from build123d import *

# Parameters (mm, degrees)
BOSS_EXTRUDE1_DEPTH                                 = 12
SHELL1_T                                            = -2.5
FILLET2_R                                           = 8
SKETCH5_R                                           = 1.5
BOSS_EXTRUDE3_DEPTH                                 = 9.5
FILLET5_R                                           = 4
CSK_FOR_M4_COUNTERSUNK_FLAT_HEAD_SCREW1_D           = 4.5
CSK_FOR_M4_COUNTERSUNK_FLAT_HEAD_SCREW1_CSINK_D     = 9.4
CSK_FOR_M4_COUNTERSUNK_FLAT_HEAD_SCREW1_CSINK_ANGLE = 90
CSK_FOR_M4_COUNTERSUNK_FLAT_HEAD_SCREW2_D           = 4.5
CSK_FOR_M4_COUNTERSUNK_FLAT_HEAD_SCREW2_CSINK_D     = 9.4
CSK_FOR_M4_COUNTERSUNK_FLAT_HEAD_SCREW2_CSINK_ANGLE = 90


with BuildPart() as part:
    # Sketch1 → Boss-Extrude1 (new body)
    with BuildSketch(Plane.XZ.offset(-76.724152422)):
        with BuildLine():
            Line((110.259063934, 82.346126643), (10.232808146, 82.346126643))
            ThreePointArc((10.232808146, 82.346126643), (4.41063977, 84.859565296), (2.246887156, 90.820537791))
            Line((2.246887156, 90.820537791), (13.35579753, 277.820529099))
            ThreePointArc((13.35579753, 277.820529099), (15.855157174, 283.168286326), (21.341718521, 285.346117951))
            Line((21.341718521, 285.346117951), (99.259600005, 285.346117951))
            ThreePointArc((99.259600005, 285.346117951), (104.747858971, 283.166686096), (107.245796332, 277.815871333))
            Line((107.245796332, 277.815871333), (118.24526026, 90.815880025))
            ThreePointArc((118.24526026, 90.815880025), (116.079632079, 84.857867678), (110.259063934, 82.346126643))
        make_face()
    extrude(amount=BOSS_EXTRUDE1_DEPTH)

    # Shell1
    shell1_openings = [part.faces().sort_by_distance(p)[0] for p in [
        (60.272055657, 76.724152422, 180.004596884),
    ]]
    offset(amount=SHELL1_T, openings=shell1_openings, kind=Kind.INTERSECTION)

    # Fillet2
    fillet2_edges = [part.edges().sort_by_distance(p)[0] for p in [
        (104.747858971, 64.724152422, 283.166686096),
        (60.300659263, 64.724152422, 285.346117951),
        (15.855157174, 64.724152422, 283.168286326),
        (7.801342343, 64.724152422, 184.320533445),
        (4.41063977, 64.724152422, 84.859565296),
        (60.24593604, 64.724152422, 82.346126643),
        (116.079632079, 64.724152422, 84.857867678),
        (112.745528296, 64.724152422, 184.315875679),
    ]]
    fillet(fillet2_edges, radius=FILLET2_R)

    # Sketch5 → Boss-Extrude3 (add)
    # profile 1 of 4: a face of its own
    with BuildSketch(Plane(origin=(0, 76.724152422, 0), x_dir=(1, 0, 0), z_dir=(0, 1, 0))):
        with BuildLine():
            Line((104.888526891, -275.315871333), (102.195926429, -275.157490782))
            ThreePointArc((102.195926429, -275.157490782), (98.472168712, -276.511008395), (96.902330565, -280.148863486))
            Line((96.902330565, -280.148863486), (96.902330565, -282.846117951))
            Line((96.902330565, -282.846117951), (99.259600005, -282.846117951))
            ThreePointArc((99.259600005, -282.846117951), (103.032778044, -281.34775855), (104.75010998, -277.669073401))
            Line((104.75010998, -277.669073401), (104.888526891, -275.315871333))
        make_face()
        with Locations(Location((100.902330565, -279.088314379, 0), (0, 0, 270))):
            Circle(SKETCH5_R, mode=Mode.SUBTRACT)
    # profile 2 of 4: a face of its own
    with BuildSketch(Plane(origin=(0, 76.724152422, 0), x_dir=(1, 0, 0), z_dir=(0, 1, 0))):
        with BuildLine():
            Line((18.401104149, -275.160761929), (15.711690126, -275.320529099))
            Line((15.711690126, -275.320529099), (15.85139784, -277.672275615))
            ThreePointArc((15.85139784, -277.672275615), (17.569707595, -281.348858709), (21.341718521, -282.846117951))
            Line((21.341718521, -282.846117951), (23.697611116, -282.846117951))
            Line((23.697611116, -282.846117951), (23.697611116, -280.151962548))
            ThreePointArc((23.697611116, -280.151962548), (22.126711958, -276.513107313), (18.401104149, -275.160761929))
        make_face()
        with Locations(Location((19.697611116, -279.090793629, 0), (0, 0, 270))):
            Circle(SKETCH5_R, mode=Mode.SUBTRACT)
    # profile 3 of 4: a face of its own
    with BuildSketch(Plane(origin=(0, 76.724152422, 0), x_dir=(1, 0, 0), z_dir=(0, 1, 0))):
        with BuildLine():
            Line((14.990438495, -84.846126643), (10.232808146, -84.846126643))
            ThreePointArc((10.232808146, -84.846126643), (6.230067388, -86.574115717), (4.742487465, -90.672284307))
            Line((4.742487465, -90.672284307), (4.990438495, -94.846126643))
            Line((4.990438495, -94.846126643), (14.990438495, -94.846126643))
            Line((14.990438495, -94.846126643), (14.990438495, -84.846126643))
        make_face()
        with Locations(Location((10.232808146, -90.346126643, 0), (0, 0, 270))):
            Circle(SKETCH5_R, mode=Mode.SUBTRACT)
    # profile 4 of 4: a face of its own
    with BuildSketch(Plane(origin=(0, 76.724152422, 0), x_dir=(1, 0, 0), z_dir=(0, 1, 0))):
        with BuildLine():
            Line((105.501426671, -84.821111223), (105.506954269, -94.821109695))
            Line((105.506954269, -94.821109695), (115.506952742, -94.815582097))
            Line((115.506952742, -94.815582097), (115.752596601, -90.641603341))
            ThreePointArc((115.752596601, -90.641603341), (114.262751603, -86.544257652), (110.259056293, -84.818481396))
            Line((110.259056293, -84.818481396), (105.501426671, -84.821111223))
        make_face()
        with Locations(Location((110.259063934, -90.346126643, 0), (0, 0, 270))):
            Circle(SKETCH5_R, mode=Mode.SUBTRACT)
    extrude(amount=-BOSS_EXTRUDE3_DEPTH)

    # Fillet5
    fillet5_edges = [part.edges().sort_by_distance(p)[0] for p in [
        (14.990438495, 71.974152422, 94.846126643),
        (105.506954269, 71.974152422, 94.821109695),
    ]]
    fillet(fillet5_edges, radius=FILLET5_R)

    # CSK for M4 Countersunk Flat Head Screw1 (through all)
    with Locations(Plane(origin=(0, 64.724152422, 0), x_dir=(-1, 0, 0), z_dir=(0, -1, 0))):
        with Locations((-10.232808146, -90.346126643), (-110.259063934, -90.346126643)):
            CounterSinkHole(CSK_FOR_M4_COUNTERSUNK_FLAT_HEAD_SCREW1_D / 2, CSK_FOR_M4_COUNTERSUNK_FLAT_HEAD_SCREW1_CSINK_D / 2, counter_sink_angle=CSK_FOR_M4_COUNTERSUNK_FLAT_HEAD_SCREW1_CSINK_ANGLE)

    # CSK for M4 Countersunk Flat Head Screw2 (through all)
    with Locations(Plane(origin=(0, 64.724152422, 0), x_dir=(-1, 0, 0), z_dir=(0, -1, 0))):
        with Locations((-100.902330565, -279.088314379), (-19.697611116, -279.090793629)):
            CounterSinkHole(CSK_FOR_M4_COUNTERSUNK_FLAT_HEAD_SCREW2_D / 2, CSK_FOR_M4_COUNTERSUNK_FLAT_HEAD_SCREW2_CSINK_D / 2, counter_sink_angle=CSK_FOR_M4_COUNTERSUNK_FLAT_HEAD_SCREW2_CSINK_ANGLE)


solid = part.part
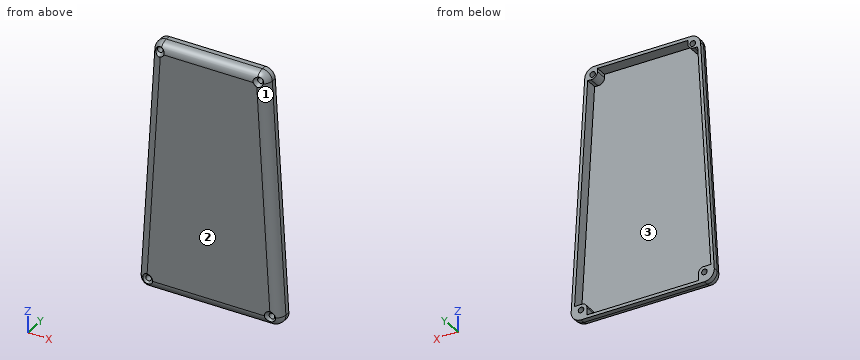
Source: CAD feature listing. Evaluate the final solid. Frame: model axes, mm. Face numbers are marked on the shaded views. Round coordinates to 2 decimals unless told otherwise and drop trailing zeros. Loops run counter-clockwise (first coordinate to the right, second up) from the corner with the lowest first, then second, coordinate; pieces in that order, holes last. Notation, with made-up numbers: (62.25, 27.5) - (80.25, 27.5) arc R17 cw to (80.25, 35.5) - close; hole circle Ø10 at (42.25, -34.75). An arc over 180 degrees is marked (long way). Write item = value, one per line. Start each with the question number.
(1) Section query A-A, the plane x = 69.5. Output: boundary loops of the cut face in (y, z), plus the area to 3 significant figures.
(2) Pull-direction query (X, two-part tool) for the marked faces 1, 2 and 3; classes: +X half, -X half, draft (parallel to the pull), parting line (faces both ways), or undercut.
(3) Ray query, line 1 along Z through (x, y) = (74.5, 74.5); line 2 along Z through (x, y) = (19, 75.5); line 3 along Y through (x, z) = (89, 162.5). Return the intervals inside material, ascending. Write a range as from..to.
(4) Pin query (flat end, axial travel): pin 1 (1.5 mm diameter, centred on y = 74.5, z = 244.5, fed in from +X); pin 2 (0.8 mm diameter, centred on y = 70, z = 281.5, fed in from +X); pin 3 (5 mm diameter, centred on x = 91, y = 69, fed in from -Z); pin 4 (2.5 mm diameter, centred on x = 100.9, z = 279.09, fed in from -Y). Return the tip coordinate at first contact, or that it passes through.
Conclusion:
q1.outline = (64.72, 90.35) arc R8 ccw to (72.72, 82.35) - (76.72, 82.35) - (76.72, 84.85) - (67.22, 84.85) - (67.22, 282.85) - (76.72, 282.85) - (76.72, 285.35) - (72.72, 285.35) arc R8 ccw to (64.72, 277.35) - close
q1.area = 528 mm2
q2.face_1 = +X half
q2.face_2 = draft
q2.face_3 = undercut
q3.line_1 = 82.35..84.85, 282.85..285.35
q3.line_2 = 82.35..84.85, 275.16..276.95, 281.23..285
q3.line_3 = 64.72..67.22
q4.pin_1 = 109.25
q4.pin_2 = 105.83
q4.pin_3 = 82.44
q4.pin_4 = through
